```python
from build123d import *

# Parameters (mm, degrees)
F3_D     = 5
F4_R     = 0.25
F5_DEPTH = 0.2
F6_R     = 0.25
F7_DEPTH = 0.2


with BuildPart() as f1:
    # F0 (on Front) → F1 (revolve)
    with BuildSketch(Plane.XZ):
        Polygon((-3.628851, 6.336789), (-4.628851, 6.336789), (-4.628851, 1.336789), (-2.128851, 1.336789), (-2.128851, -2.663211), (5.871149, -2.663211), (5.871149, 1.336789), (8.371149, 1.336789), (8.371149, 6.336789), (7.371149, 6.336789), (7.371149, 3.386789), (-3.628851, 3.386789), align=None)
    revolve(axis=Axis((1.871149, 0, -2.663211), (1, 0, 0)))

    # F3 (through all)
    with Locations(Plane(origin=(-2.128851, 0, 0), x_dir=(0, -1, 0), z_dir=(-1, 0, 0))):
        with Locations((0, -2.663211)):
            Hole(F3_D / 2)

    # F4 (on face) → F5 (cut)
    with BuildSketch(Plane.YZ.offset(8.371149)):
        with Locations((-6.479844, -3.203344)):
            Circle(F4_R)
    extrude(amount=-F5_DEPTH, mode=Mode.SUBTRACT)

    # F6 (on face) → F7 (cut)
    with BuildSketch(Plane(origin=(-4.628851, 0, 0), x_dir=(0, -1, 0), z_dir=(-1, 0, 0))):
        with Locations((-6.352625, -3.346852)):
            Circle(F6_R)
    extrude(amount=-F7_DEPTH, mode=Mode.SUBTRACT)


solid = f1.part
```
Geometry check sheet. Reference: the model listing, model coordinates, mm. A direction names the side the tool comes from. Give positions to 0.01 mm unless a question says otherwise; leave off trailing zeros. Order: outer loops, then holes, each group sorted by start corner. A loop starts at its lowest first (then second) coordinate and runs counter-clockwise, first axis right, second up. Notation, with made-up numbers: (46, 85) -> (81, 85) arc R12 cw to (81, 98) -> close; hole circle Ø3 at (74.25, -28.5). An arc over 180 degrees is marked (long way). Write each question's results on one line, items separated by ' | '. Start each with the question number.
(1) Scan lines: line 1 (Z direction, x = -0.5, y = 0); line 2 (X direction, y = 5.25, z = -8); line 3 (Z direction, x = -4.05, y = 0). Record each from-to range of solid material in increasing order.
(2) Sectioned sample at C-C (z = 2). Enter the section's corners in (x, y).
(3) Sectioned sample at A-A (y = 0). Enter the section's corners in (x, z), plus the area to 3 significant figures.
(4) Sectioned sample at B-B (z = -9.25). Enter the section's corners in (x, y), plus the area to 3 significant figures.
(5) Sectioned sample at D-D (x = 7). Enter the section's corners in (y, z), plus the area to 3 significant figures.
(6) Access from +Z, -Z, +X, -X, +Y, -Y to the whole of each face (thin tool, end or side, straight path). Record for faces 1 (the face through (5.871, 3, -3)), 2 (the face through (-3.36, 3.55, -0.82)), 3 (the face through (8.371, 2, -7)), 4 (the face through (-4.136, -8.923, -3.835)), 5 (the face through (-3.629, 6, -5)).
(7) Mould release check, pull along Z, two halves, no side actions. Record for faces 6 (the face through (7.864, -8.923, -3.835)), 7 (the face through (7.371, 6, -1)), 8 (the face through (7.14, 3.55, -0.82)), 9 (the face through (1.927, -0.542, -5.104)): pulls with the +Z half, pulls with the -Z half, needs draft (parallel to the pull), parting line crosses it, or undercut.
(8) Gauge pin test, flat ends, axial feed: P1, Ø2.5, axis at y = -1.5, z = -2.5, coming from the +X side; P2, Ø3, axis at x = 6.5, y = 1.5, coming from the -Z side; P3, Ø3, axis at x = 2.5, z = -0.5, coming from the +Y side; P4, Ø2.5, axis at y = 0.5, z = -3.5, coming from the -X side. Record the tip position at first contact, or that the pin passes through.
Answer below:
1) line 1: -8.71 to -5.16, -0.16 to 3.39 | line 2: -4.63 to -3.63, 7.37 to 8.37 | line 3: -11.66 to -6.66, 1.34 to 6.34
2) outline: (-4.63, -7.7) -> (-3.63, -7.7) -> (-3.63, -3.85) -> (7.37, -3.85) -> (7.37, -7.7) -> (8.37, -7.7) -> (8.37, 7.7) -> (7.37, 7.7) -> (7.37, 3.85) -> (-3.63, 3.85) -> (-3.63, 7.7) -> (-4.63, 7.7) -> close
3) outline: (-4.63, -11.66) -> (-3.63, -11.66) -> (-3.63, -8.71) -> (7.37, -8.71) -> (7.37, -11.66) -> (8.37, -11.66) -> (8.37, -6.66) -> (5.87, -6.66) -> (5.87, -5.16) -> (-2.13, -5.16) -> (-2.13, -6.66) -> (-4.63, -6.66) -> close; (-4.63, 1.34) -> (-2.13, 1.34) -> (-2.13, -0.16) -> (5.87, -0.16) -> (5.87, 1.34) -> (8.37, 1.34) -> (8.37, 6.34) -> (7.37, 6.34) -> (7.37, 3.39) -> (-3.63, 3.39) -> (-3.63, 6.34) -> (-4.63, 6.34) -> close | area: 89.1 mm2
4) outline: (-4.63, -6.13) -> (-3.63, -6.13) -> (-3.63, 6.13) -> (-4.63, 6.13) -> close; (7.37, -6.13) -> (8.37, -6.13) -> (8.37, 6.13) -> (7.37, 6.13) -> close | area: 24.5 mm2
5) outline: circle Ø12.1 at (0, -2.66); hole circle Ø8 at (0, -2.66) | area: 64.7 mm2
6) face 1: +X | face 2: -X | face 3: +Z, -Z, +X, +Y, -Y | face 4: +X, -X | face 5: none
7) face 6: parting line crosses it | face 7: needs draft | face 8: undercut | face 9: undercut
8) P1: x = 5.87 | P2: z = -11.66 | P3: y = 6.01 | P4: through
